```python
from build123d import *

# Parameters (mm, degrees)
F0_R     = 5.3361283698
F1_DEPTH = 25


with BuildPart() as f1:
    # F0 (on Top) → F1 (new body)
    with BuildSketch(Plane.XY):
        with BuildLine():
            ThreePointArc((14.9163241405, 52.7680086499), (14.8401902708, 54.171918287), (14.6126816385, 55.5593614236))
            ThreePointArc((14.6126816385, 55.5593614236), (2.4097380818, 65.741419961), (-10.5058992859, 56.4800777855))
            ThreePointArc((-10.5058992859, 56.4800777855), (0.0584840327, 39.9221055948), (14.9163241405, 52.7680086499))
        make_face()
        with Locations((1.9342003872, 52.7680086499)):
            Circle(F0_R, mode=Mode.SUBTRACT)
        with BuildLine():
            ThreePointArc((-25.1224026689, 7.4964106405), (-12.8838755219, 22.8328062201), (6.5711412686, 25.3801377218))
            Line((6.5711412686, 25.3801377218), (22.1448177539, 21.3479756675))
            Line((22.1448177539, 21.3479756675), (14.6126816385, 55.5593614236))
            ThreePointArc((14.6126816385, 55.5593614236), (14.8401902708, 54.171918287), (14.9163241405, 52.7680086499))
            ThreePointArc((14.9163241405, 52.7680086499), (0.0584840327, 39.9221055948), (-10.5058992859, 56.4800777855))
            Line((-10.5058992859, 56.4800777855), (-25.1224026689, 7.4964106405))
        make_face()
        with BuildLine():
            ThreePointArc((6.5711412686, 25.3801377218), (18.8746968967, 18.1955243235), (25.6038070106, 5.6370519701))
            Line((25.6038070106, 5.6370519701), (22.1448177539, 21.3479756675))
            Line((22.1448177539, 21.3479756675), (6.5711412686, 25.3801377218))
        make_face()
        with BuildLine():
            ThreePointArc((6.5711412686, -25.3801377218), (20.7317018594, -16.0476735499), (26.2170038019, 0))
            ThreePointArc((26.2170038019, 0), (26.0632537693, 2.8351527833), (25.6038070106, 5.6370519701))
            ThreePointArc((25.6038070106, 5.6370519701), (18.8746968967, 18.1955243235), (6.5711412686, 25.3801377218))
            ThreePointArc((6.5711412686, 25.3801377218), (-12.8838755219, 22.8328062201), (-25.1224026689, 7.4964106405))
            ThreePointArc((-25.1224026689, 7.4964106405), (-18.8746968967, -18.1955243235), (6.5711412686, -25.3801377218))
        make_face()
        with BuildLine():
            ThreePointArc((56.0573402856, 12.5677247968), (39.8213218542, 0), (56.0573402856, -12.5677247968))
            ThreePointArc((56.0573402856, -12.5677247968), (63.0693600951, -7.9464795272), (65.7855693607, 0))
            ThreePointArc((65.7855693607, 0), (63.0693600951, 7.9464795272), (56.0573402856, 12.5677247968))
        make_face()
        with Locations((52.8034456074, 0)):
            Circle(F0_R, mode=Mode.SUBTRACT)
        with BuildLine():
            ThreePointArc((25.6038070106, 5.6370519701), (26.0632537693, 2.8351527833), (26.2170038019, 0))
            ThreePointArc((26.2170038019, 0), (20.7317018594, -16.0476735499), (6.5711412686, -25.3801377218))
            Line((6.5711412686, -25.3801377218), (56.0573402856, -12.5677247968))
            ThreePointArc((56.0573402856, -12.5677247968), (39.8213218542, 0), (56.0573402856, 12.5677247968))
            Line((56.0573402856, 12.5677247968), (22.1448177539, 21.3479756675))
            Line((22.1448177539, 21.3479756675), (25.6038070106, 5.6370519701))
        make_face()
    extrude(amount=F1_DEPTH)


solid = f1.part
```
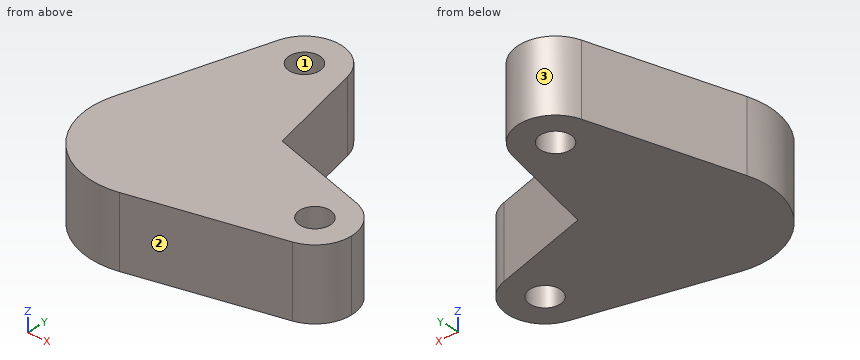
Source: CAD feature listing. Evaluate the final solid. Frame: model axes, mm. Face numbers are marked on the shaded views. Round coordinates to 2 decimals unless told otherwise and drop trailing zeros. Loops run counter-clockwise (first coordinate to the right, second up) from the corner with the lowest first, then second, coordinate; pieces in that order, holes last.
1. Section query D-D on x = 24. Output: boundary loops of the cut face in (y, z).
2. Section query C-C on y = -11.5. Output: boundary loops of the cut face in (x, z), and give its area (3 significant figures).
3. Mould query, pull axis Y, two halves, no side actions, for the marked faces 1, 2 and 3. Classes: released by +Y, released by -Y, zero draft, split by the parting line, or undercut.
4. Ray query, L1, parallel to Y at x = 51, z = 1; L2, parallel to Y at x = 48, z = 24.25; L3, parallel to X at y = 49, z = 15.5. Return the intervals inside material, ascending.
5. Section query A-A on x = -2. Output: boundary loops of the cut face in (y, z).
6. Contact query for flat-ended pins moving along their axis: pin 1 (2 mm diameter, centred on x = 48, z = 13, fed in from -Y); pin 2 (4 mm diameter, centred on x = 10, z = 11.5, fed in from -Y); pin 3 (8 mm diameter, centred on y = 35, z = 8.5, fed in from -X). Output: stop coordinate, or through.
7. Section query B-B on z = 2. Output: boundary loops of the cut face in (x, y), and give its area (3 significant figures).
Answers below:
1. outline: (-20.87, 0) - (20.87, 0) - (20.87, 25) - (-20.87, 25) - close
2. outline: (-23.56, 0) - (58.83, 0) - (58.83, 25) - (-23.56, 25) - close
2. area: 2,060 mm2
3. face 1: undercut
3. face 2: released by -Y
3. face 3: released by +Y
4. L1: y = -13.88 to -5.02, 5.02 to 13.88
4. L2: y = -14.65 to -2.32, 2.32 to 14.65
4. L3: x = -12.74 to -1.84, 5.71 to 16.06
5. outline: (-26.14, 0) - (49.16, 0) - (49.16, 25) - (-26.14, 25) - close; (56.37, 0) - (65.14, 0) - (65.14, 25) - (56.37, 25) - close
6. pin 1: stops at y = -14.91
6. pin 2: stops at y = -25.01
6. pin 3: stops at x = -18.11
7. outline: (-25.12, 7.5) arc R26.22 ccw to (6.57, -25.38) - (56.06, -12.57) arc R12.98 ccw to (56.06, 12.57) - (22.14, 21.35) - (14.61, 55.56) arc R12.98 ccw to (-10.51, 56.48) - close; hole circle Ø10.67 at (1.93, 52.77); hole circle Ø10.67 at (52.8, 0)
7. area: 4,580 mm2
